Can you work these out from the model? Positions are in its coordinate system, mm. A direction names the side the tool comes from. Give positions to 0.01 mm unless a question says otherwise; leave off trailing zeros. Loops run counter-clockwise (first coordinate to the right, second up) from the corner with the lowest first, then second, coordinate; pieces in that order, holes last. Notation, with made-up numbers: (33.5, 62.5) - (58.5, 62.5) arc R25 cw to (58.5, 101.5) - close; hole circle Ø7 at (20.25, 71). An arc over 180 degrees is marked (long way). Answer as a JSON object with one key per item and string values. Group by question number.
Item 1: Suppose I cut it at D-D on z = -35. Write out the boundary of the cut face in (x, y).
Item 2: Will these pins go through, and if not, where does the flat tip stop? pin 1 (2 mm diameter, centred on x = 7, y = 6.5, fed in from +Z); pin 2 (2 mm diameter, centred on x = 0, y = 4, fed in from -Z); pin 3 (10 mm diameter, centred on x = -37, z = -47.5, fed in from -Y); pin 4 (3 mm diameter, centred on x = -0.5, y = 5, fed in from -Z).
Item 3: Which directions (+Z, -Z, +X, -X, +Y, -Y) give clear straight access to the entire face, cutting with the end or side of a thin tool? Please do faces 5 (the flat face through (0, 0, -50)), 6 (the flat face through (49, 4, -11.5)), 7 (the flat face through (0, 4, -49.99)), 8 (the flat face through (46.674, 3.944, -8.745)), 9 (the flat face through (-47.8, 3.9, -5)).
Item 4: Please list where these lines run through material, in increasing order: L1, parallel to Y at x = 0, z = -51 (3 decimals); L2, parallel to Y at x = 49.47, z = -6.5; L3, parallel to X at y = 0.75, z = -38.
Item 5: Suppose I cut it at B-B on x = 0. Write out the boundary of the cut face in (y, z) (3 decimals), and give its area (3 significant figures).
Item 6: Suppose I cut it at A-A on y = 4. Write out the boundary of the cut face in (x, z) (3 decimals), and give its area (3 significant figures).
Item 7: Suppose I cut it at C-C on z = -24. Write out the boundary of the cut face in (x, y), and give its area (3 significant figures).
Item 8: Thinking about a two-plate mould opening in X: for faces 1 (the cylindrical face through (0.656, 1.047, -51.465)), 2 (the flat face through (-2, 1, -52.5)), 3 (the flat face through (-46.7, 3.9, -8.9)), 4 (the cylindrical face through (37.93, 3.94, -37.02)), which applies, pulls with the +X half, pulls with the -X half, needs draft (parallel to the pull), parting line crosses it, or undercut?
from build123d import *

# Parameters (mm, degrees)
BOSS_EXTRUDE1_DEPTH = 8
SKETCH4_R           = 3.025
CUT_EXTRUDE3_DEPTH  = 2.1
SKETCH5_R           = 1.45
CUT_EXTRUDE4_DEPTH  = 6.5
SKETCH6_R           = 1.75
CUT_EXTRUDE5_DEPTH  = 0.41


with BuildPart() as part:
    # Sketch1 → Boss-Extrude1 (new body)
    with BuildSketch(Plane(origin=(0, 0, 0), x_dir=(1, 0, 0), z_dir=(0, 1, 0))):
        with BuildLine():
            Line((52.763623833, 5), (46.013623833, 5))
            Line((46.013623833, 5), (47.353145997, 12.596807697))
            ThreePointArc((47.353145997, 12.596807697), (0, 49), (-47.353145997, 12.596807697))
            Line((-47.353145997, 12.596807697), (-46.013623833, 5))
            Line((-46.013623833, 5), (-52.763623833, 5))
            ThreePointArc((-52.763623833, 5), (-38.273476153, 36.66252887), (-7.262919523, 52.5))
            Line((-7.262919523, 52.5), (7.262919523, 52.5))
            ThreePointArc((7.262919523, 52.5), (38.273476153, 36.66252887), (52.763623833, 5))
        make_face()
    extrude(amount=BOSS_EXTRUDE1_DEPTH)

    # Sketch4 → Cut-Extrude3 (cut)
    with BuildSketch(Plane(origin=(0, 0, -52.5), x_dir=(-1, 0, 0), z_dir=(0, 0, -1))):
        with Locations((0, 4)):
            Circle(SKETCH4_R)
    extrude(amount=-CUT_EXTRUDE3_DEPTH, mode=Mode.SUBTRACT)

    # Sketch5 → Cut-Extrude4 (cut)
    with BuildSketch(Plane.XY.offset(-5)):
        with Locations((-49.47, 4)):
            Circle(SKETCH5_R)
    cut_extrude4 = extrude(amount=-CUT_EXTRUDE4_DEPTH, mode=Mode.SUBTRACT)

    # Mirror1: Cut-Extrude4 across plane
    add(cut_extrude4.mirror(Plane(origin=(0, 0, 0), x_dir=(0, 0, 1), z_dir=(1, 0, 0))), mode=Mode.SUBTRACT)

    # Sketch6 → Cut-Extrude5 (cut)
    with BuildSketch(Plane(origin=(0, 0, -50.4), x_dir=(-1, 0, 0), z_dir=(0, 0, -1))):
        with Locations((0, 4)):
            Circle(SKETCH6_R)
    extrude(amount=-CUT_EXTRUDE5_DEPTH, mode=Mode.SUBTRACT)


solid = part.part
Worked out:
{
 "1": {"outline": "(-39.8, 0) - (-34.29, 0) - (-34.29, 8) - (-39.8, 8) - close; (34.29, 0) - (39.8, 0) - (39.8, 8) - (34.29, 8) - close"},
 "2": {"pin 1": "stops at z = -48.34", "pin 2": "stops at z = -49.99", "pin 3": "passes through", "pin 4": "stops at z = -50.4"},
 "3": {"face 5": "+Z, -Z, +X, -X, -Y", "face 6": "+Z", "face 7": "-Z", "face 8": "+Y, -Y", "face 9": "+Z, +X, -X, +Y, -Y"},
 "4": {"L1": "y = 0 to 0.975, 7.025 to 8", "L2": "y = 0 to 2.55, 5.45 to 8", "L3": "x = -36.95 to -30.94, 30.94 to 36.95"},
 "5": {"outline": "(0, -52.5) - (0.975, -52.5) - (0.975, -50.4) - (2.25, -50.4) - (2.25, -49.99) - (5.75, -49.99) - (5.75, -50.4) - (7.025, -50.4) - (7.025, -52.5) - (8, -52.5) - (8, -49) - (0, -49) - close", "area": "13.9 mm2"},
 "6": {"outline": "(-52.764, -5) arc R53 ccw to (-7.263, -52.5) - (-3.025, -52.5) - (-3.025, -50.4) - (-1.75, -50.4) - (-1.75, -49.99) - (1.75, -49.99) - (1.75, -50.4) - (3.025, -50.4) - (3.025, -52.5) - (7.263, -52.5) arc R53 ccw to (52.764, -5) - (50.92, -5) - (50.92, -11.5) - (48.02, -11.5) - (48.02, -5) - (46.014, -5) - (47.353, -12.597) arc R49 cw to (-47.353, -12.597) - (-46.014, -5) - (-48.02, -5) - (-48.02, -11.5) - (-50.92, -11.5) - (-50.92, -5) - close", "area": "566 mm2"},
 "7": {"outline": "(-47.25, 0) - (-42.72, 0) - (-42.72, 8) - (-47.25, 8) - close; (42.72, 0) - (47.25, 0) - (47.25, 8) - (42.72, 8) - close", "area": "72.6 mm2"},
 "8": {"face 1": "undercut", "face 2": "needs draft", "face 3": "undercut", "face 4": "pulls with the +X half"}
}
